Source: CAD feature listing. Evaluate the final solid. Frame: model axes, mm. Face numbers are marked on the shaded views. A direction names the side the tool comes from. Round coordinates to 2 decimals unless told otherwise and drop trailing zeros. Loops run counter-clockwise (first coordinate to the right, second up) from the corner with the lowest first, then second, coordinate; pieces in that order, holes last. Notation, with made-up numbers: (23.5, 45) -> (37.5, 45) arc R5 ccw to (37.5, 54) -> close; hole circle Ø4 at (65.25, 72.5). An arc over 180 degrees is marked (long way). Put each result on its own line as item: value. Start each with the question number.
1. Cut plane A-A (y = 0). Return the cut outline in (x, z), then the cut area to 3 significant figures.
2. Cut plane D-D (x = -5). Return the cut outline in (y, z), then the cut area to 3 significant figures.
3. Set-up query: the marked faces 1, 2 and 3. Return all of +Z, -Z, +X, -X, +Y, -Y with unobstructed straight access to the full face (end or side cutting, diameter ignored); none if empty.
4. Material intervals for L1, parallel to X at y = 0, z = 4.75; L2, parallel to X at y = 0, z = 8.5; L3, parallel to Z at x = -4.25, y = 8.75, sorted ascending.
5. Draft query along X for the marked faces 4, 5 and 6. Return one class per face: pulls with the +X half, pulls with the -X half, needs draft (parallel to the pull), parting line crosses it, or undercut.
6. Cut plane B-B (x = 3.5). Return the cut outline in (y, z), then the cut area to 3 significant figures.
7. Cut plane C-C (z = 5). Return the cut outline in (x, y), then the cut area to 3 significant figures.
8. Contact query for flat-ended pins moving along their axis: pin 1 (4 mm diameter, centred on x = -2, y = -8, fed in from -Z); pin 2 (1 mm diameter, centred on x = 8, z = 4.5, fed in from +Y); pin 3 (4 mm diameter, centred on y = -4.5, z = 1.5, fed in from +X); pin 4 (6.5 mm diameter, centred on y = -7, z = 5.5, fed in from -X). Output: stop coordinate, or through.
```python
from build123d import *

# Parameters (mm, degrees)
F0_R      = 10.5
F1_DEPTH  = 14
F2_R      = 10.5
F2_R_2    = 6.5
F3_DEPTH  = 6
F4_R      = 4.5
F5_DEPTH  = 14.001
F6_W      = 2.713612
F6_H      = 7.583218
F7_DEPTH  = 14.001
F9_DEPTH  = 6.75
F10_W     = 22.774708
F10_H     = 11.08392
F11_DEPTH = 6.75


with BuildPart() as f1:
    # F0 (on Top) → F1 (new body)
    with BuildSketch(Plane.XY):
        Circle(F0_R)
    extrude(amount=F1_DEPTH)

    # F2 (on face) → F3 (cut)
    with BuildSketch(Plane.XY.offset(14)):
        Circle(F2_R)
        Circle(F2_R_2, mode=Mode.SUBTRACT)
    extrude(amount=-F3_DEPTH, mode=Mode.SUBTRACT)

    # F4 (on face) → F5 (cut, through all)
    with BuildSketch(Plane.XY.offset(14)):
        Circle(F4_R)
    extrude(amount=-F5_DEPTH, mode=Mode.SUBTRACT)

    # F6 (on Top) → F7 (cut, through all)
    with BuildSketch(Plane.XY):
        with Locations((0, -7.369267)):
            Rectangle(F6_W, F6_H)
    extrude(amount=F7_DEPTH, mode=Mode.SUBTRACT)

    # F8 (on face) → F9 (cut)
    with BuildSketch(Plane.XY.offset(14)):
        with BuildLine():
            ThreePointArc((10.981682, 0.794768), (0, 11.010404), (-10.981682, 0.794768))
            Line((-10.981682, 0.794768), (-6.469861, 0.794768))
            ThreePointArc((-6.469861, 0.794768), (0, 6.518493), (6.469861, 0.794768))
            Line((6.469861, 0.794768), (10.981682, 0.794768))
        make_face()
    extrude(amount=-F9_DEPTH, mode=Mode.SUBTRACT)

    # F10 (on face) → F11 (cut)
    with BuildSketch(Plane.XY.offset(14)):
        with Locations((-0.604641, 6.395375)):
            Rectangle(F10_W, F10_H)
    extrude(amount=-F11_DEPTH, mode=Mode.SUBTRACT)


solid = f1.part
```
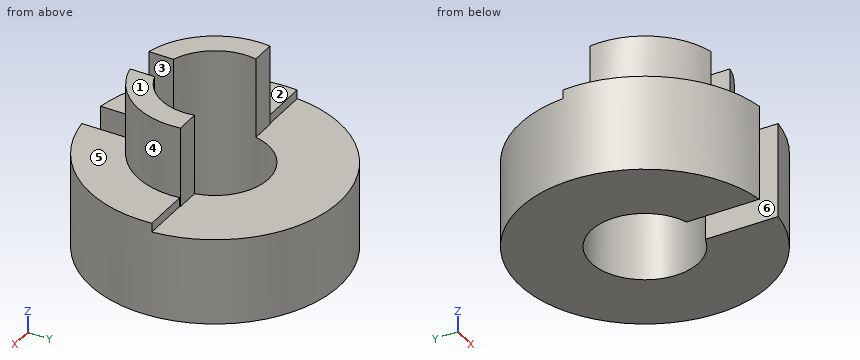
Solution:
1. outline: (-10.5, 0) -> (-4.5, 0) -> (-4.5, 14) -> (-6.5, 14) -> (-6.5, 8) -> (-10.5, 8) -> close; (4.5, 0) -> (10.5, 0) -> (10.5, 8) -> (6.5, 8) -> (6.5, 14) -> (4.5, 14) -> close
1. area: 120 mm^2
2. outline: (-9.23, 0) -> (9.23, 0) -> (9.23, 7.25) -> (0.85, 7.25) -> (0.85, 14) -> (-4.15, 14) -> (-4.15, 8) -> (-9.23, 8) -> close
2. area: 171 mm^2
3. face 1: +Z, +X, -X, +Y, -Y
3. face 2: +Z, -X, -Y
3. face 3: +Z, -Z, -Y
4. L1: x = -10.5 to -4.5, 4.5 to 10.5
4. L2: x = -6.5 to -4.5, 4.5 to 6.5
4. L3: z = 0 to 7.25
5. face 4: pulls with the +X half
5. face 5: needs draft
5. face 6: undercut
6. outline: (-9.9, 0) -> (-2.83, 0) -> (-2.83, 14) -> (-5.48, 14) -> (-5.48, 8) -> (-9.9, 8) -> close; (2.83, 0) -> (9.9, 0) -> (9.9, 7.25) -> (2.83, 7.25) -> close
6. area: 124 mm^2
7. outline: (-1.36, -10.41) -> (-1.36, -4.29) arc R4.5 cw (long way) to (1.36, -4.29) -> (1.36, -10.41) arc R10.5 ccw (long way) to start
7. area: 266 mm^2
8. pin 1: stops at z = 0
8. pin 2: stops at y = 7.35
8. pin 3: stops at x = 10.2
8. pin 4: stops at x = -9.81
